from build123d import *

# Parameters (mm, degrees)
BOSS_EXTRUDE1_DEPTH = 11
SKETCH2_W           = 1
SKETCH2_H           = 11
BOSS_EXTRUDE2_DEPTH = 9.2
SKETCH3_R           = 2.1
CUT_EXTRUDE1_DEPTH  = 10


with BuildPart() as part:
    # Sketch1 → Boss-Extrude1 (new body)
    with BuildSketch(Plane.XY):
        with BuildLine():
            Line((0, 0), (0, 2.4))
            ThreePointArc((0, 2.4), (3, 5.4), (0, 8.4))
            Line((0, 8.4), (0, 10.8))
            Line((0, 10.8), (10.5, 10.8))
            Line((10.5, 10.8), (10.5, 0))
            Line((10.5, 0), (0, 0))
        make_face()
    extrude(amount=BOSS_EXTRUDE1_DEPTH)

    # Sketch2 → Boss-Extrude2 (add)
    with BuildSketch(Plane(origin=(0, 10.8, 0), x_dir=(1, 0, 0), z_dir=(0, 1, 0))):
        with Locations((10, -5.5)):
            Rectangle(SKETCH2_W, SKETCH2_H)
    extrude(amount=BOSS_EXTRUDE2_DEPTH)

    # Sketch3 → Cut-Extrude1 (cut)
    with BuildSketch(Plane.ZY.offset(-9.5)):
        with Locations((5.5, 16)):
            Circle(SKETCH3_R)
    extrude(amount=-CUT_EXTRUDE1_DEPTH, mode=Mode.SUBTRACT)


solid = part.part
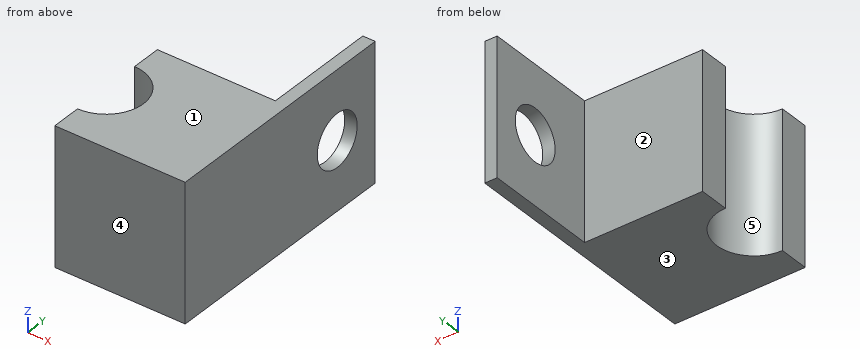
Geometry check sheet. Reference: the model listing, model coordinates, mm. Face numbers are marked on the shaded views. A direction names the side the tool comes from. Coordinates: 2 decimals unless noted, no trailing zeros. Order: outer loops, then holes, each group sorted by start corner. A loop starts at its lowest first (then second) coordinate and runs counter-clockwise, first axis right, second up. Notation, with made-up numbers: (56.25, 37) - (95.25, 37) arc R28 cw to (95.25, 75) - close; hole circle Ø8 at (76.25, -31.75). An arc over 180 degrees is marked (long way). Answer in a Markdown table with one row per item. Add a question column.
1) Cross-section at C-C, the plane z = 10. Record the cut outline in (x, y), then the cut area to 3 significant figures.
2) Cross-section at A-A, the plane z = 5.5. Record the cut outline in (x, y), then the cut area to 3 significant figures.
3) Cross-section at D-D, the plane y = 5.4. Record the cut outline in (x, z).
4) Set-up check for the marked faces 1 and 2: record each of +Z, -Z, +X, -X, +Y, -Y from which the full face is reachable in a straight line by a thin tool's end or side.
5) Release check for a two-part mould opening along Y. For the marked faces 3, 4 and 5 record: +Y half, -Y half, draft (parallel to the pull), parting line (faces both ways), or undercut.
6) Cross-section at B-B, the plane y = 16. Record the cut outline in (x, z).
7) Material ranges on line 1 along Y through (x, z) = (9.9, 5.5); line 2 along Y through (x, z) = (6, 3.25); line 3 along Y through (x, z) = (2.75, 8.75), recorded low to high. Write a range as [from, to].
8) Gauge pin test, flat end, axial feed: P1, Ø3, axis at x = 3, z = 3.5, coming from the +Y side. Record the tip position at first contact, or that the pin passes through.
Check result:
| question | item | result |
|---|---|---|
| 1 | outline | (0, 0) - (10.5, 0) - (10.5, 20) - (9.5, 20) - (9.5, 10.8) - (0, 10.8) - (0, 8.4) arc R3 cw to (0, 2.4) - close |
| 1 | area | 108 mm² |
| 2 | outline | (0, 0) - (10.5, 0) - (10.5, 13.9) - (9.5, 13.9) - (9.5, 10.8) - (0, 10.8) - (0, 8.4) arc R3 cw to (0, 2.4) - close; (9.5, 18.1) - (10.5, 18.1) - (10.5, 20) - (9.5, 20) - close |
| 2 | area | 104 mm² |
| 3 | outline | (3, 0) - (10.5, 0) - (10.5, 11) - (3, 11) - close |
| 4 | face 1 | +Z, +X, -X, +Y, -Y |
| 4 | face 2 | +Z, -Z, -X, +Y |
| 5 | face 3 | draft |
| 5 | face 4 | -Y half |
| 5 | face 5 | undercut |
| 6 | outline | (9.5, 0) - (10.5, 0) - (10.5, 3.4) - (9.5, 3.4) - close; (9.5, 7.6) - (10.5, 7.6) - (10.5, 11) - (9.5, 11) - close |
| 7 | line 1 | y = [0, 13.9], [18.1, 20] |
| 7 | line 2 | y = [0, 10.8] |
| 7 | line 3 | y = [0, 4.2], [6.6, 10.8] |
| 8 | P1 | stops at y = 10.8 |
